For this review, take the finished solid that the model builds, in its own axes (mm). A direction names the side the tool comes from. Give positions to 0.01 mm unless a question says otherwise; leave off trailing zeros. Write each loop counter-clockwise with the first axis right and the second up, starting at its lowest first coordinate (ties: lowest second). Pieces come first, ordered by that corner, then holes. Notation, with made-up numbers: (-8.75, 34.5) -> (31.25, 34.5) arc R22 ccw to (31.25, 61.5) -> close; hole circle Ø8 at (22, 15.5). An arc over 180 degrees is marked (long way). Answer as CSV lines item,"result".
```python
from build123d import *

# Parameters (mm, degrees)
SKETCH_W        = 1200
SKETCH_H        = 650
PAD_DEPTH       = 50
SKETCH001_W     = 30
SKETCH001_H     = 30
POCKET_DEPTH    = 1100
SKETCH002_W     = 30
SKETCH002_H     = 30
POCKET001_DEPTH = 1200
SKETCH003_R     = 20
POCKET002_DEPTH = 45
SKETCH004_R     = 10
POCKET003_DEPTH = 45


with BuildPart() as part:
    # Sketch → Pad (new body)
    with BuildSketch(Plane.XY):
        Polygon((0, 0), (0, 1100), (50, 1100), (50, 950), (1250, 950), (1250, 1100), (1300, 1100), (1300, 0), (1250, 0), (1250, 200), (50, 200), (50, 0), align=None)
        with Locations((650, 575)):
            Rectangle(SKETCH_W, SKETCH_H, mode=Mode.SUBTRACT)
    extrude(amount=PAD_DEPTH)

    # Sketch001 (on Face2 of Pad) → Pocket (cut)
    with BuildSketch(Plane.XZ):
        with Locations((25, 25)):
            Rectangle(SKETCH001_W, SKETCH001_H)
        with Locations((1275, 25)):
            Rectangle(SKETCH001_W, SKETCH001_H)
    extrude(amount=-POCKET_DEPTH, mode=Mode.SUBTRACT)

    # Sketch002 (on Face19 of Pocket) → Pocket001 (cut)
    with BuildSketch(Plane.YZ.offset(50)):
        with Locations((225, 25)):
            Rectangle(SKETCH002_W, SKETCH002_H)
        with Locations((925, 25)):
            Rectangle(SKETCH002_W, SKETCH002_H)
    extrude(amount=POCKET001_DEPTH, mode=Mode.SUBTRACT)

    # Sketch003 (on Face5 of Pocket001) → Pocket002 (cut)
    with BuildSketch(Plane.XY.offset(50)):
        with Locations((25, 1050)):
            Circle(SKETCH003_R)
        with Locations((1275, 1050)):
            Circle(SKETCH003_R)
    extrude(amount=-POCKET002_DEPTH, mode=Mode.SUBTRACT)

    # Sketch004 (on Face5 of Pocket002) → Pocket003 (cut)
    with BuildSketch(Plane.XY.offset(50)):
        with Locations((25, 50)):
            Circle(SKETCH004_R)
    extrude(amount=-POCKET003_DEPTH, mode=Mode.SUBTRACT)


solid = part.part
```
Q1. Add section C-C (x = 1275). Write out the cut boundary in (y, z).
Answer block:
outline,"(0, 0) -> (1100, 0) -> (1100, 10) -> (1070, 10) -> (1070, 5) -> (1030, 5) -> (1030, 10) -> (0, 10) -> close; (0, 40) -> (1030, 40) -> (1030, 50) -> (0, 50) -> close; (1070, 40) -> (1100, 40) -> (1100, 50) -> (1070, 50) -> close"
Q2. Draft analysis for pull direction Z (two halves, no side actions). For faces 1 (the flat face through (50, 101, 25)), 2 (the flat face through (1290, 511, 25)), 3 (the flat face through (642, 225, 40)), 4 (the flat face through (701, 227, 0)), state which applies: released by +Z, released by -Z, zero draft, split by the parting line, or undercut.
Answer block:
face 1,"zero draft"
face 2,"undercut"
face 3,"undercut"
face 4,"released by -Z"
Q3. Add section A-A (x = 266). Write out the cut boundary in (y, z).
Answer block:
outline,"(200, 0) -> (250, 0) -> (250, 50) -> (200, 50) -> close; (900, 0) -> (950, 0) -> (950, 50) -> (900, 50) -> close; hole (210, 10) -> (240, 10) -> (240, 40) -> (210, 40) -> close; hole (910, 10) -> (940, 10) -> (940, 40) -> (910, 40) -> close"
Q4. For faces 5 (the flat face through (1260, 511, 25)), 6 (the flat face through (642, 925, 40)), 7 (the flat face through (1250, 99, 25)), 8 (the flat face through (25, 1050, 5)), list the 3-axis set-ups (+Z, -Z, +X, -X, +Y, -Y) from which the entire face can be reached by the end or side of a thin tool; tool diameter is ignored.
Answer block:
face 5,"+Y, -Y"
face 6,"none"
face 7,"+Z, -Z, -Y"
face 8,"+Z"
Q5. Add section D-D (z = 29.5). State how many separate pieces and enclosed holes the cut face has, plus the area to 3 significant figures.
Answer block:
separate pieces,"3"
enclosed holes,"3"
area,"91,600 mm2"
Q6. To check wall thickness, follow probe 1 along X at (y, z) = (557, 34); probe 2 along Y at (x, z) = (25, 44); probe 3 along Y at (x, z) = (482, 15.5). State the ranges of each line that lie inside material, in increasing order. Write a range as [from, to].
Answer block:
probe 1,"x = [0, 10], [40, 50], [1250, 1260], [1290, 1300]"
probe 2,"y = [0, 40], [60, 1030], [1070, 1100]"
probe 3,"y = [200, 210], [240, 250], [900, 910], [940, 950]"
Q7. Clearance check with flat-ended pins moving along their axes: pin 1 (24 mm diameter, centred on x = 460, z = 26, fed in from +Y); pin 2 (1.5 mm diameter, centred on x = 335, z = 23, fed in from -Y); pin 3 (18 mm diameter, centred on x = 25, y = 50, fed in from +Z). State where each tip first meets the part, or that it passes through.
Answer block:
pin 1,"stops at y = 950"
pin 2,"stops at y = 200"
pin 3,"stops at z = 5"
Q8. Add section B-B (y = 310). Write out the cut boundary in (x, z).
Answer block:
outline,"(0, 0) -> (50, 0) -> (50, 50) -> (0, 50) -> close; (1250, 0) -> (1300, 0) -> (1300, 50) -> (1250, 50) -> close; hole (10, 10) -> (40, 10) -> (40, 40) -> (10, 40) -> close; hole (1260, 10) -> (1290, 10) -> (1290, 40) -> (1260, 40) -> close"
